Autodesk Inventor part; units mm, degrees
ref_plane "YZ Plane" through (0, 0, 0) normal (1, 0, 0) x (0, 1, 0)
ref_plane "XZ Plane" through (0, 0, 0) normal (0, 1, 0) x (-1, 0, 0)
ref_plane "XY Plane" through (0, 0, 0) normal (0, 0, 1) x (1, 0, 0)
sketch "Sketch1" plane through (0, 0, 0) normal (0, 1, 0) x (-1, 0, 0)
  line L0 (24.5, 21.15) -> (-24.5, 21.15)
  line L1 (-24.5, 21.15) -> (-24.5, -21.15)
  line L2 (-24.5, -21.15) -> (24.5, -21.15)
  line L3 (24.5, -21.15) -> (24.5, 21.15)
  line L4 (24.5, 21.15) -> (-24.5, -21.15) construction
  line L5 (-24.5, 21.15) -> (24.5, -21.15) construction
  circle A0 centre (0, 0) radius 12
  circle A1 centre (15.5, -15.5) radius 1.5
  line L6 (0, 0) -> (0, -30.8544) construction
  line L7 (0, 0) -> (-33.5596, 0) construction
  circle A2 centre (15.5, 15.5) radius 1.5
  circle A3 centre (-15.5, -15.5) radius 1.5
  circle A4 centre (-15.5, 15.5) radius 1.5
  dimension "d0" = 49
  dimension "d1" = 42.3
  dimension "d2" = 24
  dimension "d3" = 15.5
  dimension "d4" = 3
  dimension "d5" = 15.5
  dimension "d8" = 31
  dimension "d11" = 31
extrude "Extrusion1" add sketch "Sketch1" along normal blind 3
sketch "Sketch2" plane through (0, 0, 0) normal (0, -1, 0) x (1, 0, 0)
  line L0 (-24.5, 21.15) -> (24.5, 21.15)
  line L1 (24.5, -21.15) -> (-24.5, -21.15)
  line L2 (24.5, 21.15) -> (21.5, 21.15)
  line L3 (21.5, 21.15) -> (21.5, -21.15)
  line L4 (21.5, -21.15) -> (24.5, -21.15)
  line L5 (24.5, -21.15) -> (24.5, 21.15)
  point P0 (0, 0)
  dimension "d16" = 3
extrude "Extrusion2" add sketch "Sketch2" along normal blind 48
sketch "Sketch3" plane through (24.5, 3, 21.15) normal (1, 0, 0) x (0, 0, -1)
  line L0 (0, -51) -> (42.3, -51)
  line L1 (0, -51) -> (42.3, -51)
  line L2 (42.3, -51) -> (42.3, -48)
  line L3 (42.3, -48) -> (0, -48)
  line L4 (0, -48) -> (0, -51)
  point P0 (21.15, -3)
  dimension "d19" = 3
extrude "Extrusion3" add sketch "Sketch3" along normal blind 10
sketch "Sketch4" plane through (24.5, -45, 21.15) normal (0, 1, 0) x (1, 0, 0)
  circle A0 centre (5.5, 36.65) radius 1.5
  circle A1 centre (-9, 36.65) radius 1.5
  line L0 (-24.5, 21.15) -> (15.0504, 21.15) construction
  circle A2 centre (5.5, 5.65) radius 1.5
  dimension "d22" = 3
  dimension "d23" = 30
extrude "Extrusion4" cut sketch "Sketch4" against normal through all contours A0 | A2
mirror "Mirror1" about plane through (0, 0, 0) normal (1, 0, 0)
equation "\"d5\" = d3"
properties part number "Motor_cage_3DPrint"
Design review of the part built by this model. Coordinates are the model's own, in mm. A direction names the side the tool comes from. Coordinates: 2 decimals unless noted, no trailing zeros. Order: outer loops, then holes, each group sorted by start corner. A loop starts at its lowest first (then second) coordinate and runs counter-clockwise, first axis right, second up. Notation, with made-up numbers: M 7.5,39.25 L 45.5,39.25 A14 ccw 45.5,61.25 Z; hole C 9,24 d4. An arc over 180 degrees is marked long. Answer as a JSON object with one key per item and string values. Group by question number.
1) Mouldability with a two-part tool opening along X and no side actions: class faces 1 (the flat face through (21.5, -24, 0)), 2 (the cylindrical face through (-28.5, -46.48, -15.43)), 3 (the flat face through (-29, -45, 0)), 4 (the flat face through (-24.5, -21, 0)) as pulls with the +X half, pulls with the -X half, needs draft (parallel to the pull), parting line crosses it, or undercut.
2) Tool access review of faces 5 (the flat face through (29, -45, 0)), 6 (the flat face through (-21.5, -24, 0)), 7 (the flat face through (11.2, 3, 5)): name each direction out of +Z, -Z, +X, -X, +Y, -Y from which nothing blocks a thin tool from reaching the whole face with its end or side.
3) Add section D-D, the plane y = -19. Write out the cut boundary in (x, z).
4) Wall thickness on L1, parallel to X at y = -47.15, z = -15.5; L2, parallel to Z at x = -15.5, y = 1.5; L3, parallel to X at y = 0.9, z = -15.5: over which ranges is each line inside the solid? List them lowest first.
5) For pin 1 (3.5 mm diameter, centred on x = -15.5, z = -15.5, fed in from -Y); pin 2 (12.5 mm diameter, centred on y = -26, z = 4.5, fed in from +X); pin 3 (2 mm diameter, centred on y = -27, z = -14.5, fed in from -X); pin 4 (1.8 mm diameter, centred on x = -30, z = -15.5, fed in from -Y), all flat-tipped, find the tip position at first contact; note any pin that passes through.
6) Add section A-A, the plane z = -15.5. Write out the cut boundary in (x, y), then the cut area to 3 significant figures.
7) Add section B-B, the plane x = 30. Write out the cut boundary in (y, z).
8) Add section C-C, the plane z = 0. Write out the cut boundary in (x, y), then the cut area to 3 significant figures.
Computed values:
{
 "1": {"face 1": "undercut", "face 2": "undercut", "face 3": "needs draft", "face 4": "pulls with the -X half"},
 "2": {"face 5": "+Z, -Z, +X, +Y", "face 6": "+Z, -Z, -Y", "face 7": "+Z, -Z, +X, -X, +Y"},
 "3": {"outline": "M -24.5,-21.15 L -21.5,-21.15 L -21.5,21.15 L -24.5,21.15 Z; M 21.5,-21.15 L 24.5,-21.15 L 24.5,21.15 L 21.5,21.15 Z"},
 "4": {"L1": "x = -34.5 to -31.5, -28.5 to -21.5, 21.5 to 28.5, 31.5 to 34.5", "L2": "z = -21.15 to -17, -14 to 14, 17 to 21.15", "L3": "x = -24.5 to -17, -14 to 14, 17 to 24.5"},
 "5": {"pin 1": "stops at y = 0", "pin 2": "stops at x = 24.5", "pin 3": "stops at x = -24.5", "pin 4": "passes through"},
 "6": {"outline": "M -34.5,-48 L -31.5,-48 L -31.5,-45 L -34.5,-45 Z; M -28.5,-48 L -21.5,-48 L -21.5,0 L -17,0 L -17,3 L -24.5,3 L -24.5,-45 L -28.5,-45 Z; M -14,0 L 14,0 L 14,3 L -14,3 Z; M 17,0 L 21.5,0 L 21.5,-48 L 28.5,-48 L 28.5,-45 L 24.5,-45 L 24.5,3 L 17,3 Z; M 31.5,-48 L 34.5,-48 L 34.5,-45 L 31.5,-45 Z", "area": "459 mm^2"},
 "7": {"outline": "M -48,-21.15 L -45,-21.15 L -45,-17 L -48,-17 Z; M -48,-14 L -45,-14 L -45,14 L -48,14 Z; M -48,17 L -45,17 L -45,21.15 L -48,21.15 Z"},
 "8": {"outline": "M -34.5,-48 L -21.5,-48 L -21.5,0 L -12,0 L -12,3 L -24.5,3 L -24.5,-45 L -34.5,-45 Z; M 12,0 L 21.5,0 L 21.5,-48 L 34.5,-48 L 34.5,-45 L 24.5,-45 L 24.5,3 L 12,3 Z", "area": "423 mm^2"}
}
